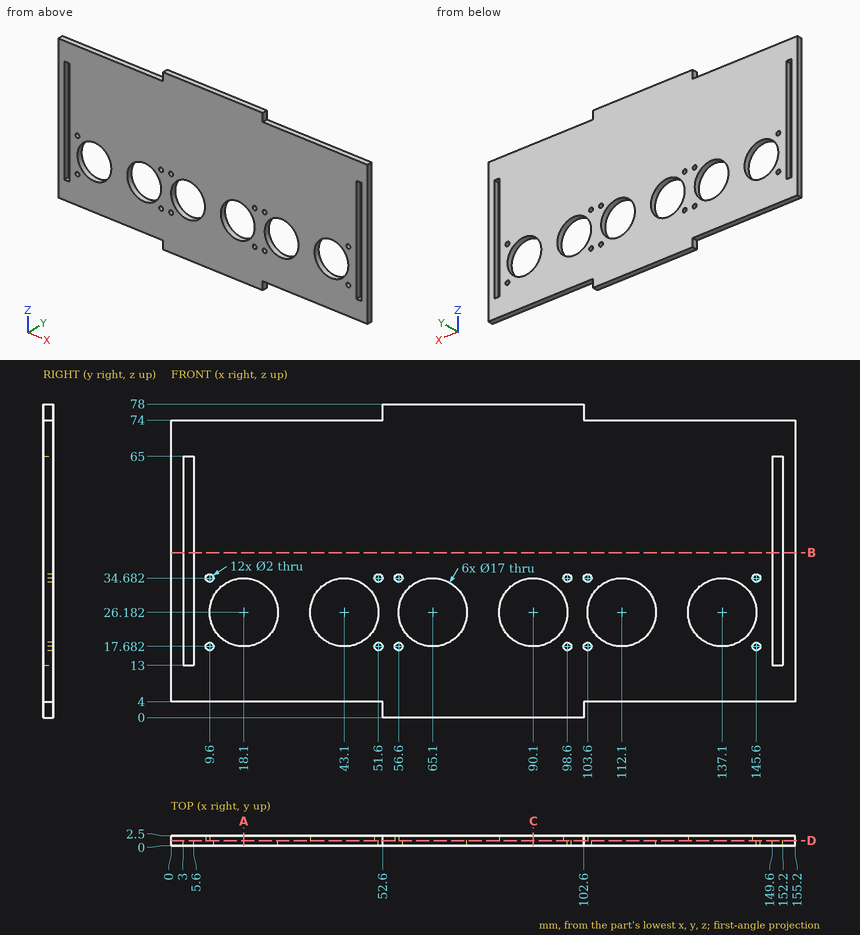
Study the drawing (mm; zero at the part's minimum x, y, z) and answer. Give positions to 0.01 mm unless a question says otherwise; leave off trailing zeros. Write each loop counter-clockwise with the first axis right and the second up, starting at its lowest first coordinate (ties: lowest second). Pieces come first, ordered by that corner, then holes. Notation, with made-up numbers: (28.5, 85) -> (65.5, 85) arc R18 ccw to (65.5, 100) -> close; hole circle Ø11 at (7, -10.75). An arc over 180 degrees is marked (long way). Answer as a JSON object with one key per item and string values. Group by question number.
1) Each of these flat-tipped pins is pushed along its axis until it touches: P1, Ø0.8, axis at x = 151, y = 1.5, coming from the -Z side; P2, Ø0.8, axis at y = 1, z = 2, coming from the -X side. Where does it stop, or does it pass through?
2) Consider L1, parallel to X at y = 1.1, z = 56; L2, parallel to Z at x = 112, y = 2.35; L3, parallel to Z at x = 124, y = 0.25. Determine where each line is inside the solid, lowest interval first. Write a range as from..to.
3) Find section D-D (y = 1.25). Count the separate pieces of the cut face and the enclosed holes in it, and give its area (3 significant figures).
4) Find section A-A (x = 18.1). Write down the section's boundary in (y, z).
5) Find section C-C (x = 90.1). Write down the section's boundary in (y, z).
6) Find section B-B (z = 41). Write down the section's boundary in (x, y).
Values follow:
{
 "1": {"P1": "stops at z = 4", "P2": "stops at x = 52.6"},
 "2": {"L1": "x = 0..3, 5.6..149.6, 152.2..155.2", "L2": "z = 4..17.68, 34.68..74", "L3": "z = 4..74"},
 "3": {"separate pieces": "1", "enclosed holes": "20", "area": "9,590 mm2"},
 "4": {"outline": "(0, 4) -> (2.5, 4) -> (2.5, 17.68) -> (0, 17.68) -> close; (0, 34.68) -> (2.5, 34.68) -> (2.5, 74) -> (0, 74) -> close"},
 "5": {"outline": "(0, 0) -> (2.5, 0) -> (2.5, 17.68) -> (0, 17.68) -> close; (0, 34.68) -> (2.5, 34.68) -> (2.5, 78) -> (0, 78) -> close"},
 "6": {"outline": "(0, 0) -> (3, 0) -> (3, 2.5) -> (0, 2.5) -> close; (5.6, 0) -> (149.6, 0) -> (149.6, 2.5) -> (5.6, 2.5) -> close; (152.2, 0) -> (155.2, 0) -> (155.2, 2.5) -> (152.2, 2.5) -> close"}
}
